Read the model definition and answer for the solid it produces. Units are mm, in the model's axes. Face numbers are marked on the shaded views. A direction names the side the tool comes from. Give positions to 0.01 mm unless a question says otherwise; leave off trailing zeros. Write each loop counter-clockwise with the first axis right and the second up, starting at its lowest first coordinate (ties: lowest second). Pieces come first, ordered by that corner, then holes. Notation, with made-up numbers: M -7,-21 L 27,-21 A22 ccw 27,-1 Z; hole C 36,28 d4. An arc over 180 degrees is marked long. Put each result on its own line as item: value.
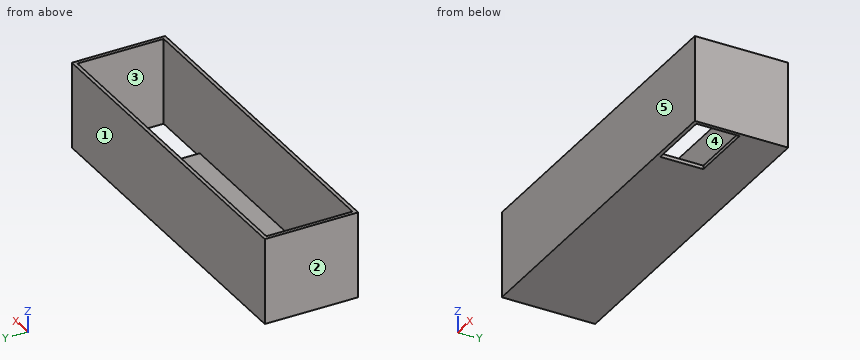
from build123d import *

# Parameters (mm, degrees)
SKETCH1_W           = 609.6
SKETCH1_H           = 165.1
BOSS_EXTRUDE1_DEPTH = 152.4
SHELL1_T            = -6.35
SKETCH4_W           = 114.3
SKETCH4_H           = 76.2
CUT_EXTRUDE1_DEPTH  = 6.35


with BuildPart() as part:
    # Sketch1 → Boss-Extrude1 (new body)
    with BuildSketch(Plane.XY):
        with Locations((0, 82.55)):
            Rectangle(SKETCH1_W, SKETCH1_H)
    extrude(amount=-BOSS_EXTRUDE1_DEPTH)

    # Shell1
    shell1_openings = [part.faces().sort_by_distance(p)[0] for p in [
        (0, 82.55, 0),
    ]]
    offset(amount=SHELL1_T, openings=shell1_openings, kind=Kind.INTERSECTION)

    # Sketch4 → Cut-Extrude1 (cut)
    with BuildSketch(Plane(origin=(0, 0, -152.4), x_dir=(-1, 0, 0), z_dir=(0, 0, -1))):
        with Locations((-241.3, 44.45)):
            Rectangle(SKETCH4_W, SKETCH4_H)
    extrude(amount=-CUT_EXTRUDE1_DEPTH, mode=Mode.SUBTRACT)


solid = part.part
(1) Which of the six approach directions +Z, -Z, +X, -X, +Y, -Y give full straight-line access (tool end or side, diameter ignored) to the marked faces 4 and 5?
Result:
face 4: +Z
face 5: +Z, -Z, +X, -X, -Y
(2) Section A-A on y = 24 is taken. Determine the outline of the cut face in (x, z), and give its area (3 significant figures).
Result:
outline: M -304.8,-152.4 L 184.15,-152.4 L 184.15,-146.05 L -298.45,-146.05 L -298.45,0 L -304.8,0 Z; M 298.45,-152.4 L 304.8,-152.4 L 304.8,0 L 298.45,0 Z
area: 5,000 mm²
(3) Section B-B on z = -118.5 is taken. Determine the outline of the cut face in (x, y).
Result:
outline: M -304.8,0 L 304.8,0 L 304.8,165.1 L -304.8,165.1 Z; hole M -298.45,6.35 L 298.45,6.35 L 298.45,158.75 L -298.45,158.75 Z
(4) Section C-C on x = 222.5 is taken. Determine the outline of the cut face in (y, z).
Result:
outline: M 0,-152.4 L 6.35,-152.4 L 6.35,0 L 0,0 Z; M 82.55,-152.4 L 165.1,-152.4 L 165.1,0 L 158.75,0 L 158.75,-146.05 L 82.55,-146.05 Z
(5) Section D-D on y = 117 is taken. Determine the outline of the cut face in (x, z), and give its area (3 significant figures).
Result:
outline: M -304.8,-152.4 L 304.8,-152.4 L 304.8,0 L 298.45,0 L 298.45,-146.05 L -298.45,-146.05 L -298.45,0 L -304.8,0 Z
area: 5,730 mm²
(6) For a pull along X with two mould halves and no side action, classify the marked faces 1, 2 and 3 as +X half, -X half, draft (parallel to the pull), parting line (faces both ways), or undercut.
Result:
face 1: draft
face 2: -X half
face 3: undercut
(7) Straight lines are drawn through the part: line 1 along Y through (x, z) = (207.5, -109); line 2 along X through (y, z) = (26, -110.5). For each, find the intervals that lie inside material, in ascending order. Write a range as from..to.
Result:
line 1: y = 0..6.35, 158.75..165.1
line 2: x = -304.8..-298.45, 298.45..304.8
